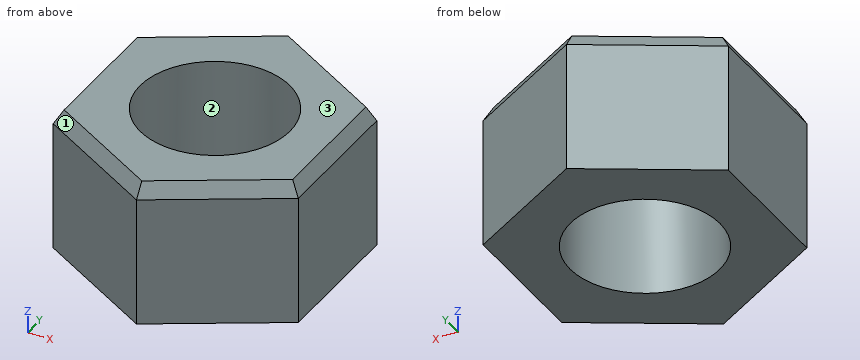
from build123d import *

# Parameters (mm, degrees)
F0_R     = 5.2
F1_DEPTH = 10
F2_SIZE2 = 0.57735
F2_SIZE  = 1


with BuildPart() as f1:
    # F0 (on Top) → F1 (new body)
    with BuildSketch(Plane.XY):
        Polygon((8.5, -4.907477), (8.5, 4.907477), (0, 9.814955), (-8.5, 4.907477), (-8.5, -4.907477), (0, -9.814955), align=None)
        Circle(F0_R, mode=Mode.SUBTRACT)
    extrude(amount=F1_DEPTH)

    # F2
    f2_edges = [f1.edges().sort_by_distance(p)[0] for p in [
        (-4.25, 7.361216, 10),
        (4.25, 7.361216, 10),
        (8.5, 0, 10),
        (4.25, -7.361216, 10),
        (-4.25, -7.361216, 10),
        (-8.5, 0, 10),
    ]]
    chamfer(f2_edges, length=F2_SIZE, length2=F2_SIZE2)


solid = f1.part
For this review, take the finished solid that the model builds, in its own axes (mm). Face numbers are marked on the shaded views. Round coordinates to 2 decimals unless told otherwise and drop trailing zeros. Order: outer loops, then holes, each group sorted by start corner. A loop starts at its lowest first (then second) coordinate and runs counter-clockwise, first axis right, second up. Notation, with made-up numbers: M 75,11 L 84,11 A12 cw 84,22 Z; hole C -19.75,28 d6. An arc over 180 degrees is marked long. Write each question's results on one line, items separated by ' | '. Start each with the question number.
1. Add section C-C (x = -5.5). State the section outline as (y, z) points.
2. Clearance check with a flat-ended pin moving along its axis: pin 1 Ø2 at (x, z) = (5.5, 6) entering from +Y. State where the tip first meets the part, or that it passes through.
3. Add section D-D (y = -6). State the section outline as (x, z) points.
4. Draft analysis for pull direction X (two halves, no side actions). For the marked faces 1, 2 and 3, state which applies: pulls with the +X half, pulls with the -X half, needs draft (parallel to the pull), parting line crosses it, or undercut.
5. Add section B-B (x = -0.75). State the section outline as (y, z) points.
6. To check wall thickness, follow L1, parallel to Y at x = 0.75, z = 7.25; L2, parallel to Y at x = 1, z = 1.5; L3, parallel to X at y = -3, z = 9. State the ranges of each line that lie inside material, in increasing order. Write a range as [from, to].
7. Add section A-A (y = 0.5). State the section outline as (x, z) points, then the cut area to 3 significant figures.
Output values:
1) outline: M -6.64,0 L 6.64,0 L 6.64,9 L 5.97,10 L -5.97,10 L -6.64,9 Z
2) pin 1: y = 7.22
3) outline: M -6.61,0 L 6.61,0 L 6.61,9 L 5.45,10 L -5.45,10 L -6.61,9 Z
4) face 1: pulls with the -X half | face 2: undercut | face 3: needs draft
5) outline: M -9.38,0 L -5.15,0 L -5.15,10 L -8.72,10 L -9.38,9 Z; M 5.15,0 L 9.38,0 L 9.38,9 L 8.72,10 L 5.15,10 Z
6) L1: [-9.38, -5.15], [5.15, 9.38] | L2: [-9.24, -5.1], [5.1, 9.24] | L3: [-8.5, -4.25], [4.25, 8.5]
7) outline: M -8.5,0 L -5.18,0 L -5.18,10 L -7.92,10 L -8.5,9 Z; M 5.18,0 L 8.5,0 L 8.5,9 L 7.92,10 L 5.18,10 Z | area: 65.9 mm^2
